Geometry: final body of the model. Coordinates: model frame, mm. Face numbers are marked on the shaded views. A direction names the side the tool comes from. Coordinates: 2 decimals unless noted, no trailing zeros. Loops run counter-clockwise (first coordinate to the right, second up) from the corner with the lowest first, then second, coordinate; pieces in that order, holes last. Notation, with made-up numbers: (-1, 89.5) -> (39, 89.5) arc R28 cw to (39, 115.5) -> close; hole circle Ø4 at (-22, 49). An arc over 180 degrees is marked (long way). One line per item, written item: value. Start each with the question number.
Item 1: Section query A-A on z = -10.25. Return loops of the section in (x, y), then the cut area to 3 significant figures.
Item 2: Mould query, pull axis Z, two halves, no side actions, for the marked faces 1, 2 and 3. Classes: +Z half, -Z half, draft (parallel to the pull), parting line (faces both ways), or undercut.
Item 3: Section query C-C on y = 2. Return loops of the section in (x, z).
Item 4: Section query B-B on x = -11.5. Return loops of the section in (y, z), then the cut area to 3 significant figures.
Item 5: Contact query for flat-ended pins moving along their axis: pin 1 Ø3 at (x, z) = (-8, 8.5) entering from +Y; pin 2 Ø2 at (y, z) = (5.5, 1) entering from +X; pin 3 Ø2 at (y, z) = (6.5, -6) entering from -X; pin 4 Ø6 at (y, z) = (6, 7.5) entering from +X. Output: stop coordinate, or through.
Item 6: Ray query, probe 1 along Z at (x, y) = (1.5, 5.25); probe 2 along X at (y, z) = (10, -8.75); probe 3 along X at (y, z) = (10.25, -2.75). Return the intervals inside material, ascending. Write a range as from..to.
Item 7: Set-up query: the marked faces 4 and 5. Return all of +Z, -Z, +X, -X, +Y, -Y with unobstructed straight access to the full face (end or side cutting, diameter ignored); none if empty.
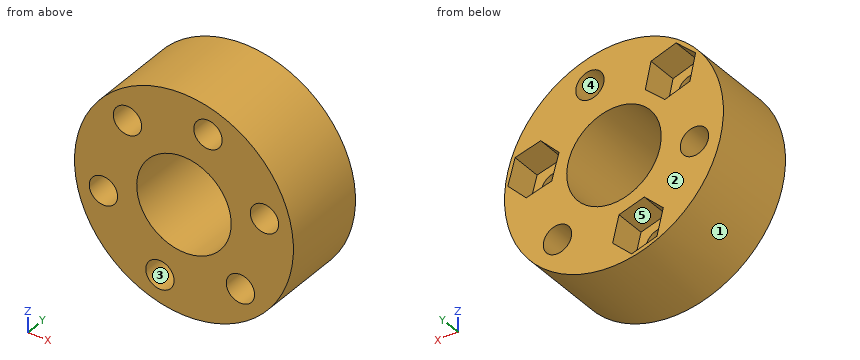
from build123d import *

# Parameters (mm, degrees)
ESQUISSE3_R             = 13.9
ESQUISSE3_R_2           = 6
ESQUISSE3_R_3           = 1.8
BOSS_EXTRU_1_DEPTH      = 11
ENL_V_MAT_EXTRU_1_DEPTH = 3.9


with BuildPart() as part:
    # Esquisse3 → Boss.-Extru.1 (new body)
    with BuildSketch(Plane(origin=(0, 0, 0), x_dir=(1, 0, 0), z_dir=(0, 1, 0))):
        with Locations(Location((0, 0, 0), (0, 0, 270))):
            Circle(ESQUISSE3_R)
        with Locations(Location((0, 0, 0), (0, 0, 270))):
            Circle(ESQUISSE3_R_2, mode=Mode.SUBTRACT)
        with Locations(Location((-3.050511372, 10.04710806, 0), (0, 0, 270))):
            Circle(ESQUISSE3_R_3, mode=Mode.SUBTRACT)
        with Locations(Location((7.175795129, 7.665374373, 0), (0, 0, 270))):
            Circle(ESQUISSE3_R_3, mode=Mode.SUBTRACT)
        with Locations(Location((10.2263065, -2.381733688, 0), (0, 0, 270))):
            Circle(ESQUISSE3_R_3, mode=Mode.SUBTRACT)
        with Locations(Location((3.050511372, -10.04710806, 0), (0, 0, 270))):
            Circle(ESQUISSE3_R_3, mode=Mode.SUBTRACT)
        with Locations(Location((-7.175795129, -7.665374373, 0), (0, 0, 270))):
            Circle(ESQUISSE3_R_3, mode=Mode.SUBTRACT)
        with Locations(Location((-10.2263065, 2.381733688, 0), (0, 0, 270))):
            Circle(ESQUISSE3_R_3, mode=Mode.SUBTRACT)
    extrude(amount=BOSS_EXTRU_1_DEPTH)

    # Esquisse4 → Enlèv. mat.-Extru.1 (cut)
    with BuildSketch(Plane(origin=(0, 11, 0), x_dir=(1, 0, 0), z_dir=(0, 1, 0))):
        Polygon((-3.859043077, 6.797552734), (-0.640579761, 7.722121401), (0.167951944, 10.971676727), (-2.241979667, 13.296663386), (-5.460442982, 12.372094719), (-6.268974687, 9.122539393), align=None)
        Polygon((12.555495262, -4.787604225), (13.474445885, -1.567532319), (11.145257124, 0.838338219), (7.897117739, 0.02413685), (6.978167116, -3.195935057), (9.307355877, -5.601805594), align=None)
        Polygon((-4.701263167, -9.921482726), (-3.984682, -6.650421008), (-6.459213962, -4.394312654), (-9.650327091, -5.409266019), (-10.366908258, -8.680327737), (-7.892376296, -10.936436091), align=None)
    extrude(amount=-ENL_V_MAT_EXTRU_1_DEPTH, mode=Mode.SUBTRACT)


solid = part.part
Reply:
1. outline: (-9.39, 0) -> (-4.84, 0) -> (-4.84, 7.1) -> (-5.99, 7.1) -> (-5.99, 11) -> (-9.39, 11) -> close; (-1.26, 0) -> (9.39, 0) -> (9.39, 11) -> (-0.01, 11) -> (-0.01, 7.1) -> (-1.26, 7.1) -> close
1. area: 158 mm²
2. face 1: parting line
2. face 2: draft
2. face 3: undercut
3. outline: circle Ø27.8 at (0, 0); hole circle Ø3.6 at (-10.23, -2.38); hole circle Ø3.6 at (-7.18, 7.67); hole circle Ø12 at (0, 0); hole circle Ø3.6 at (-3.05, -10.05); hole circle Ø3.6 at (3.05, 10.05); hole circle Ø3.6 at (7.18, -7.67); hole circle Ø3.6 at (10.23, 2.38)
4. outline: (0, -7.81) -> (11, -7.81) -> (11, -3.65) -> (0, -3.65) -> close; (0, -1.11) -> (11, -1.11) -> (11, 7.81) -> (0, 7.81) -> close
4. area: 144 mm²
5. pin 1: stops at y = 7.1
5. pin 2: stops at x = 13.9
5. pin 3: stops at x = -12.97
5. pin 4: stops at x = 13.15
6. probe 1: z = -13.82..-5.81, 5.81..9.13, 10.96..13.82
6. probe 2: x = -10.8..-5.88, -0.38..5.74, 8.61..10.8
6. probe 3: x = -13.63..-11.99, -8.46..-5.33, 5.33..13.63
7. face 4: +Y, -Y
7. face 5: +Y
